```python
from build123d import *

# Parameters (mm, degrees)
SKETCH1_R           = 11
SKETCH1_R_2         = 4
SKETCH1_R_3         = 1.75
BOSS_EXTRUDE1_DEPTH = 3.5
SKETCH1_3_R         = 5.1
SKETCH1_3_R_2       = 4
BOSS_EXTRUDE2_DEPTH = 13.5
CHAMFER1_SIZE       = 0.25


with BuildPart() as part:
    # Sketch1 → Boss-Extrude1 (new body)
    with BuildSketch(Plane(origin=(0, 0, 0), x_dir=(1, 0, 0), z_dir=(0, 1, 0))):
        Circle(SKETCH1_R)
        Circle(SKETCH1_R_2, mode=Mode.SUBTRACT)
        with Locations((0, 8.05)):
            Circle(SKETCH1_R_3, mode=Mode.SUBTRACT)
        with Locations((8.05, 0)):
            Circle(SKETCH1_R_3, mode=Mode.SUBTRACT)
        with Locations((0, -8.05)):
            Circle(SKETCH1_R_3, mode=Mode.SUBTRACT)
        with Locations((-8.05, 0)):
            Circle(SKETCH1_R_3, mode=Mode.SUBTRACT)
    extrude(amount=BOSS_EXTRUDE1_DEPTH)

    # Sketch1_3 → Boss-Extrude2 (add)
    with BuildSketch(Plane(origin=(0, 0, 0), x_dir=(1, 0, 0), z_dir=(0, 1, 0))):
        Circle(SKETCH1_3_R)
        Circle(SKETCH1_3_R_2, mode=Mode.SUBTRACT)
    extrude(amount=BOSS_EXTRUDE2_DEPTH)

    # Chamfer1
    chamfer1_edges = [part.edges().sort_by_distance(p)[0] for p in [
        (-9.8, 3.5, 0),
        (-1.75, 0, 8.05),
        (-9.8, 0, 0),
        (-1.75, 3.5, 8.05),
        (6.3, 3.5, 0),
        (-5.1, 3.5, 0),
        (-4, 13.5, 0),
        (-5.1, 13.5, 0),
        (-1.75, 3.5, -8.05),
        (-11, 3.5, 0),
        (-4, 0, 0),
        (-11, 0, 0),
        (-1.75, 0, -8.05),
        (6.3, 0, 0),
    ]]
    chamfer(chamfer1_edges, length=CHAMFER1_SIZE)


solid = part.part
```
Work out the finished part from the listing and answer in its coordinate system (mm). A direction names the side the tool comes from. Coordinates: 2 decimals unless noted, no trailing zeros. Order: outer loops, then holes, each group sorted by start corner. A loop starts at its lowest first (then second) coordinate and runs counter-clockwise, first axis right, second up. Notation, with made-up numbers: (-8.75, 15) - (26.25, 15) arc R19 ccw to (26.25, 48) - close; hole circle Ø6 at (-21, 58). An arc over 180 degrees is marked (long way). Answer as a JSON object with one key per item and string values.
1. The mould has two halves that part along Z. Classify faces 3 (the face through (-2.38, 1.73, 10.74)), 4 (the face through (-9.8, 1.73, -0.08)), 5 (the face through (2, 13.5, 4)): +Z half, -Z half, draft (parallel to the pull), parting line (faces both ways), or undercut.
Output values:
{"face 3": "parting line", "face 4": "undercut", "face 5": "draft"}
2. Find section A-A on y = 2. Determine the outline of the cut face in (x, z).
Output values:
{"outline": "circle Ø22 at (0, 0); hole circle Ø3.5 at (-8.05, 0); hole circle Ø8 at (0, 0); hole circle Ø3.5 at (0, -8.05); hole circle Ø3.5 at (0, 8.05); hole circle Ø3.5 at (8.05, 0)"}
3. Find section D-D on y = 12.5. Determine the outline of the cut face in (x, z), plus the area to 3 significant figures.
Output values:
{"outline": "circle Ø10.2 at (0, 0); hole circle Ø8 at (0, 0)", "area": "31.4 mm²"}
4. Find section B-B on z = 0. Count the separate pieces of the cut face and the enclosed holes in it, plus the area to 3 significant figures.
Output values:
{"separate pieces": "4", "enclosed holes": "0", "area": "46.0 mm²"}
5. Consider line 1 (Z direction, x = 0, y = 1.4); line 2 (X direction, y = 1.5, z = -1.25). Determine where each line is inside the solid, lowest interval first.
Output values:
{"line 1": "z = -11 to -9.8, -6.3 to -4, 4 to 6.3, 9.8 to 11", "line 2": "x = -10.93 to -9.27, -6.83 to -3.8, 3.8 to 6.83, 9.27 to 10.93"}
6. A tool of negligible diameter and unlimited length cuts with its end or side. For faces 1 (the face through (6.3, 1.73, -0.08)), 2 (the face through (2.4, 8.4, 4.5)), from which of +Z, -Z, +X, -X, +Y, -Y can it reach the whole face along a straight path? Write none if from no direction.
Output values:
{"face 1": "+Y, -Y", "face 2": "+Y"}
7. Each of these flat-tipped pins is pushed along its axis until it touches: P1, Ø8, axis at x = -5.5, y = 2.5, coming from the -Z side; P2, Ø8, axis at x = -8, y = 10, coming from the -Z side; P3, Ø5.5, axis at x = 0, z = -8.05, coming from the +Y side. Where does it stop, or does it pass through?
Output values:
{"P1": "stops at z = -10.9", "P2": "stops at z = -3.16", "P3": "stops at y = 3.55"}
